from build123d import *

# Parameters (mm, degrees)
SKETCH1_R           = 1
SKETCH1_W           = 38
SKETCH1_H           = 11
MAIN_EXTRUDE_DEPTH  = 3
WIRE_CUT_DEPTH      = 35.860436027
WIRE_CUT_DEPTH_BACK = 35.860436027
SKETCH2_R           = 1.5
FILLET1_R           = 10
FILLET2_R           = 3
FILLET3_R           = 2


with BuildPart() as part:
    # Sketch1 → Main extrude (new body)
    with BuildSketch(Plane(origin=(0, 0, 0), x_dir=(1, 0, 0), z_dir=(0, 1, 0))):
        with BuildLine():
            Line((-32, 8.5), (-32, -8.5))
            ThreePointArc((-32, -8.5), (-30.535533906, -12.035533906), (-27, -13.5))
            Line((-27, -13.5), (27, -13.5))
            ThreePointArc((27, -13.5), (30.535533906, -12.035533906), (32, -8.5))
            Line((32, -8.5), (32, 8.5))
            ThreePointArc((32, 8.5), (30.535533906, 12.035533906), (27, 13.5))
            Line((27, 13.5), (-27, 13.5))
            ThreePointArc((-27, 13.5), (-30.535533906, 12.035533906), (-32, 8.5))
        make_face()
        with Locations(Location((-21.005953225, -0.5, 0), (0, 0, 270))):
            Circle(SKETCH1_R, mode=Mode.SUBTRACT)
        with Locations(Location((20.994046775, -0.5, 0), (0, 0, 270))):
            Circle(SKETCH1_R, mode=Mode.SUBTRACT)
        Rectangle(SKETCH1_W, SKETCH1_H, mode=Mode.SUBTRACT)
    extrude(amount=MAIN_EXTRUDE_DEPTH)

    # Sketch2 → Wire cut (cut, two sides: drawn at the far end of the back side and taken through both)
    with BuildSketch(Plane(origin=(0, 3, 0), x_dir=(1, 0, 0), z_dir=(0, 1, 0)).offset(-WIRE_CUT_DEPTH_BACK)):
        with Locations((0, 5.5)):
            Circle(SKETCH2_R)
    extrude(amount=WIRE_CUT_DEPTH + WIRE_CUT_DEPTH_BACK, mode=Mode.SUBTRACT)

    # Fillet1
    fillet1_edges = [part.edges().sort_by_distance(p)[0] for p in [
        (-1.5, 1.5, -5.5),
        (1.5, 1.5, -5.5),
    ]]
    fillet(fillet1_edges, radius=FILLET1_R)

    # Fillet2
    # the kernel refuses this fillet: 3 mm, written as the material it takes off along each edge
    with BuildSketch(Plane(origin=(0, 3, -5.5), x_dir=(0.003141587485879651, 0, 0.9999950652018582), z_dir=(-0.9999950652018582, 0, 0.003141587485879651))) as fillet2_piece_1:
        with BuildLine():
            CenterArc((1.5 + FILLET2_R, -FILLET2_R), FILLET2_R, 90, 90)
            Line((1.5 + FILLET2_R, 0), (1.5, 0))
            Line((1.5, 0), (1.5, -FILLET2_R))
        make_face()
    revolve(axis=Axis((0, 3, -5.5), (0, 1, 0)), revolution_arc=359.64, mode=Mode.SUBTRACT)

    # Fillet3
    fillet3_edges = [part.edges().sort_by_distance(p)[0] for p in [
        (0, 3, 5.5),
    ]]
    fillet(fillet3_edges, radius=FILLET3_R)


solid = part.part
Work out the finished part from the listing and answer in its coordinate system (mm). A direction names the side the tool comes from. Round coordinates to 2 decimals unless told otherwise and drop trailing zeros. Loops run counter-clockwise (first coordinate to the right, second up) from the corner with the lowest first, then second, coordinate; pieces in that order, holes last. Notation, with made-up numbers: M 65.5,24 L 114.5,24 A15 ccw 114.5,37 Z; hole C -0.75,83 d3. An arc over 180 degrees is marked long. One line per question, with ' | ' between items. Start each with the question number.
(1) For a pull along Z with two mould halves and no side action, classify faces 4 (the face through (0, 1, -13.5)), 5 (the face through (-12, 1, -5.5)), 6 (the face through (-32, 1, 0)) as released by +Z, released by -Z, zero draft, split by the parting line, or undercut.
(2) Find the intervals of material crossed by line 1 (X direction, y = 1.15, z = 0.5); line 2 (X direction, y = 1.75, z = 4.25); line 3 (Z direction, x = -9, y = 0.75), in increasing order.
(3) A tool of negligible diameter and unlimited length cuts with its end or side. For faces 1 (the face through (-3.65, 1.15, -5.71)), 2 (the face through (0.27, 2.4, 6.07)), 3 (the face through (-8, 3, -6)), from which of +Z, -Z, +X, -X, +Y, -Y can it reach the whole face along a straight path? Write none if from no direction.
(4) A cutting plane is placed at B-B on z = 0.5. Write down the section's boundary in (x, y), plus the area to 3 significant figures.
(5) A cutting plane is placed at C-C on y = 1.9. Write down the section's boundary in (x, z), plus the area to 3 significant figures.
(6) A cutting plane is placed at D-D on z = 6.5. Write down the section's boundary in (x, y), plus the area to 3 significant figures.
(7) A cutting plane is placed at A-A on x = -16. Write down the section's boundary in (y, z).
Geometry check:
1) face 4: released by -Z | face 5: undercut | face 6: zero draft
2) line 1: x = -32 to -22.01, -20.01 to -19, 19 to 19.99, 21.99 to 32 | line 2: x = -32 to -19, 19 to 32 | line 3: z = -13.5 to -5.5, 5.5 to 13.5
3) face 1: +Y, -Y | face 2: +Y | face 3: +Z, -Z, +X, -X, +Y
4) outline: M -32,0 L -22.01,0 L -22.01,3 L -32,3 Z; M -20.01,0 L -19,0 L -19,3 L -20.01,3 Z; M 19,0 L 19.99,0 L 19.99,3 L 19,3 Z; M 21.99,0 L 32,0 L 32,3 L 21.99,3 Z | area: 66.0 mm²
5) outline: M -32,-8.5 A5 ccw -27,-13.5 L 27,-13.5 A5 ccw 32,-8.5 L 32,8.5 A5 ccw 27,13.5 L -27,13.5 A5 ccw -32,8.5 Z; hole C -21.01,0.5 d2; hole M -19,-5.5 L -5.68,-5.5 A10 cw -2.07,-6.17 A2.18 ccw 2.07,-6.17 A10 cw 5.68,-5.5 L 19,-5.5 L 19,5.71 L -19,5.71 Z; hole C 20.99,0.5 d2 | area: 1,270 mm²
6) outline: M -32,0 L 32,0 L 32,3 L 19,3 L 19,2.73 L -19,2.73 L -19,3 L -32,3 Z | area: 182 mm²
7) outline: M 0,-13.5 L 3,-13.5 L 3,-5.5 L 0,-5.5 Z; M 0,5.5 L 1,5.5 A2 ccw 3,7.5 L 3,13.5 L 0,13.5 Z
